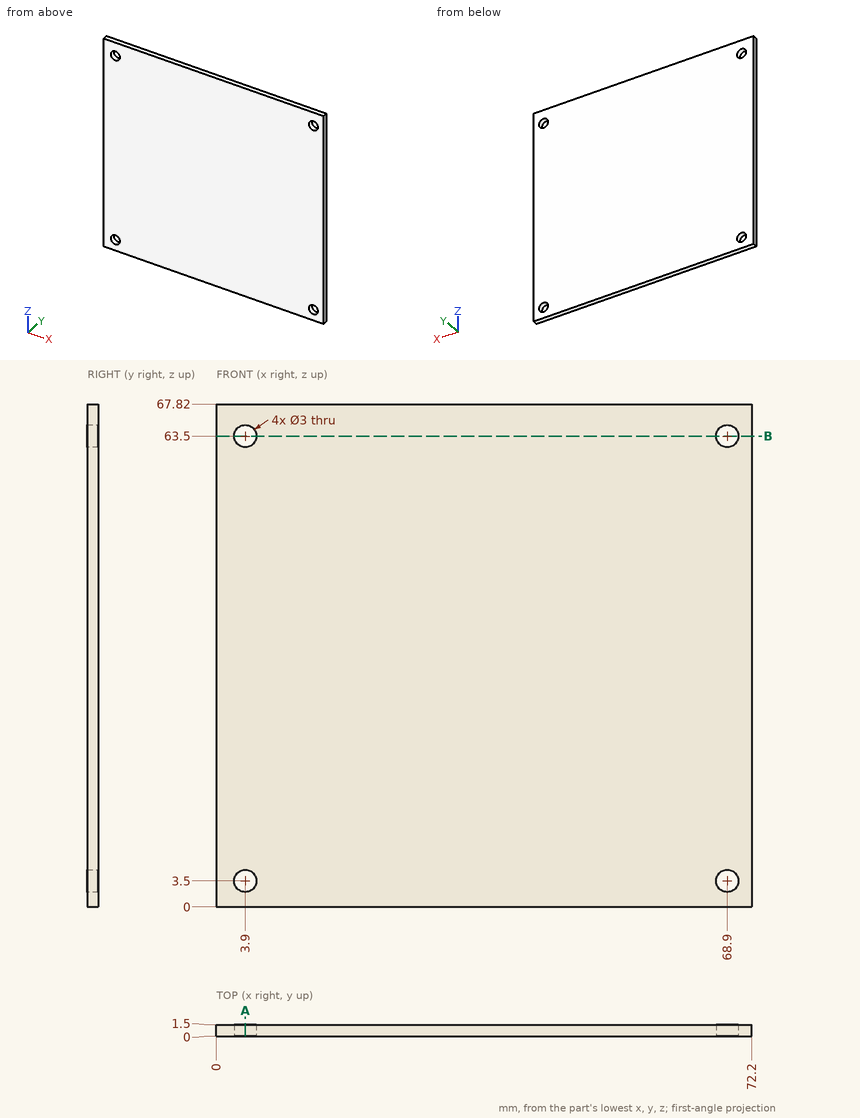
The figure shows three views and two pictorial views of one solid part (mm, origin at its lowest corner). Answer the questions. Round coordinates to 2 decimals unless told otherwise and drop trailing zeros. Loops run counter-clockwise (first coordinate to the right, second up) from the corner with the lowest first, then second, coordinate; pieces in that order, holes last. Notation, with made-up numbers: M -11.5,83.5 L 42.5,83.5 A13 ccw 42.5,87.5 Z; hole C 89,11.5 d7. An arc over 180 degrees is marked long. Use CSV: the item, a comma, the result in double quotes.
Q1. Section B-B, the plane z = 63.5 is taken. Determine the outline of the cut face in (x, y), then the cut area to 3 significant figures.
Determined:
outline,"M 0,0 L 2.4,0 L 2.4,1.5 L 0,1.5 Z; M 5.4,0 L 67.4,0 L 67.4,1.5 L 5.4,1.5 Z; M 70.4,0 L 72.2,0 L 72.2,1.5 L 70.4,1.5 Z"
area,"99.3 mm2"
Q2. This flat-tipped pin is pushed along its axis until it touches: pin 1 (1.8 mm diameter, centred on x = 3.9, z = 63.5, fed in from +Y) (3 decimals). Where does it stop, or does it pass through?
Determined:
pin 1,"through"
Q3. Section A-A, the plane x = 3.9 is taken. Determine the outline of the cut face in (y, z).
Determined:
outline,"M 0,0 L 1.5,0 L 1.5,2 L 0,2 Z; M 0,5 L 1.5,5 L 1.5,62 L 0,62 Z; M 0,65 L 1.5,65 L 1.5,67.82 L 0,67.82 Z"
Q4. Consider L1, parallel to Z at x = 68.9, y = 1.05; L2, parallel to X at y = 0.85, z = 3.5. Determine where each line is inside the solid, lowest interval first.
Determined:
L1,"0 to 2, 5 to 62, 65 to 67.82"
L2,"0 to 2.4, 5.4 to 67.4, 70.4 to 72.2"
